Work out the finished part from the listing and answer in its coordinate system (mm). A direction names the side the tool comes from. Coordinates: 2 decimals unless noted, no trailing zeros. Order: outer loops, then holes, each group sorted by start corner. A loop starts at its lowest first (then second) coordinate and runs counter-clockwise, first axis right, second up. Notation, with made-up numbers: (20.25, 12.25) -> (59.25, 12.25) arc R18 ccw to (59.25, 21.25) -> close; hole circle Ø2 at (53.5, -5.75). An arc over 180 degrees is marked (long way). Answer as CSV lines item,"result". Start each with the question number.
Item 1: For a pull along Z with two mould halves and no side action, classify faces 1 (the face through (-10, 1, 0)), 2 (the face through (-15.225, -7.133, -11.292)), 3 (the face through (-7, 0, -10)) as pulls with the +Z half, pulls with the -Z half, needs draft (parallel to the pull), parting line crosses it, or undercut.
Item 2: Straight lines are drawn through the part: L1, parallel to Y at x = -11.75, z = -9.5; L2, parallel to X at y = -4, z = -18.75 (3 decimals); L3, parallel to Y at x = -14.5, z = -2. For each, find the intervals that lie inside material, in ascending order.
Item 3: Which of the six approach directions +Z, -Z, +X, -X, +Y, -Y give full straight-line access (tool end or side, diameter ignored) to faces 4 (the face through (-15.225, -7.133, -1.132)), 5 (the face through (-14.6, -7.938, -11.4))?
Item 4: Section D-D (z = -12.5) is taken. Write down the section's boundary in (x, y) (3 decimals).
Item 5: Section C-C (x = -9.5) is taken. Write down the section's boundary in (y, z).
Item 6: Section B-B (y = -6) is taken. Write down the section's boundary in (x, z) (3 decimals).
Item 7: This flat-tipped pin is pushed along its axis until it touches: pin 1 Ø4 at (y, z) = (-6.5, -5) entering from +X (3 decimals). Where does it stop, or does it pass through?
```python
from build123d import *

# Parameters (mm, degrees)
SKETCH1_W           = 15.875
SKETCH1_H           = 20.32
BOSS_EXTRUDE1_DEPTH = 2.54
SKETCH2_W           = 2.54
SKETCH2_H           = 20.32
BOSS_EXTRUDE2_DEPTH = 6.35
SKETCH3_R           = 0.635
BOSS_EXTRUDE3_DEPTH = 1.5875


with BuildPart() as part:
    # Sketch1 → Boss-Extrude1 (new body)
    with BuildSketch(Plane(origin=(0, 0, 0), x_dir=(1, 0, 0), z_dir=(0, 1, 0))):
        with Locations((-7.9375, 10.16)):
            Rectangle(SKETCH1_W, SKETCH1_H)
    extrude(amount=BOSS_EXTRUDE1_DEPTH)

    # Sketch2 → Boss-Extrude2 (add)
    with BuildSketch(Plane.XZ):
        with Locations((-14.605, -10.16)):
            Rectangle(SKETCH2_W, SKETCH2_H)
    extrude(amount=BOSS_EXTRUDE2_DEPTH)

    # Sketch3 → Boss-Extrude3 (add)
    with BuildSketch(Plane.XZ.offset(6.35)):
        with Locations(Location((-14.605, -1.27, 0), (0, 0, 270))):
            Circle(SKETCH3_R)
        with Locations(Location((-14.605, -3.81, 0), (0, 0, 270))):
            Circle(SKETCH3_R)
        with Locations(Location((-14.605, -6.35, 0), (0, 0, 270))):
            Circle(SKETCH3_R)
        with Locations(Location((-14.605, -8.89, 0), (0, 0, 270))):
            Circle(SKETCH3_R)
        with Locations(Location((-14.605, -11.43, 0), (0, 0, 270))):
            Circle(SKETCH3_R)
        with Locations(Location((-14.605, -13.97, 0), (0, 0, 270))):
            Circle(SKETCH3_R)
        with Locations(Location((-14.605, -16.51, 0), (0, 0, 270))):
            Circle(SKETCH3_R)
        with Locations(Location((-14.605, -19.05, 0), (0, 0, 270))):
            Circle(SKETCH3_R)
    extrude(amount=BOSS_EXTRUDE3_DEPTH)


solid = part.part
```
Checked values:
1,face 1,"pulls with the +Z half"
1,face 2,"undercut"
1,face 3,"needs draft"
2,L1,"y = 0 to 2.54"
2,L2,"x = -15.875 to -13.335"
2,L3,"y = -6.35 to 2.54"
3,face 4,"-Y"
3,face 5,"+Z, -Z, +X, -X, -Y"
4,outline,"(-15.875, -6.35) -> (-13.335, -6.35) -> (-13.335, 0) -> (0, 0) -> (0, 2.54) -> (-15.875, 2.54) -> close"
5,outline,"(0, -20.32) -> (2.54, -20.32) -> (2.54, 0) -> (0, 0) -> close"
6,outline,"(-15.875, -20.32) -> (-13.335, -20.32) -> (-13.335, 0) -> (-15.875, 0) -> close"
7,pin 1,"stops at x = -13.335"
